from build123d import *

# Parameters (mm, degrees)
SKETCH_1_W               = 20
SKETCH_1_H               = 20
EXTRUDE_1_DEPTH          = 150
SKETCH_3_R               = 3.2
CUT_EXTRUDE_2_DEPTH      = 18
SKETCH_4_R               = 3.1
CUT_EXTRUDE_3_DEPTH      = 3.2
MIRROR_3_COPY_1_SKETCH_R = 3.1
MIRROR_3_COPY_1_DEPTH    = 3.2
MIRROR_4_COPY_1_SKETCH_R = 3.2
MIRROR_4_COPY_1_DEPTH    = 18
MIRROR_4_COPY_2_SKETCH_R = 3.1
MIRROR_4_COPY_2_DEPTH    = 3.2
MIRROR_4_COPY_3_SKETCH_R = 3.1
MIRROR_4_COPY_3_DEPTH    = 3.2
MIRROR_4_COPY_4_SKETCH_R = 3.1
MIRROR_4_COPY_4_DEPTH    = 3.2


with BuildPart() as part:
    # ｽｹｯﾁ1 → ﾎﾞｽ - 押し出し1 (new body)
    with BuildSketch(Plane.XY):
        Rectangle(SKETCH_1_W, SKETCH_1_H)
    extrude_1 = extrude(amount=EXTRUDE_1_DEPTH)

    # ｽｹｯﾁ3 → ｶｯﾄ - 押し出し2 (cut)
    with BuildSketch(Plane(origin=(0, 10, 0), x_dir=(1, 0, 0), z_dir=(0, 1, 0))):
        with Locations(Location((5, -5, 0), (0, 0, 270))):
            Circle(SKETCH_3_R)
    cut_extrude_2 = extrude(amount=-CUT_EXTRUDE_2_DEPTH, mode=Mode.SUBTRACT)

    # ﾐﾗｰ1: ｶｯﾄ - 押し出し2 across plane
    add(cut_extrude_2.mirror(Plane(origin=(0, 0, 0), x_dir=(0, 0, 1), z_dir=(1, 0, 0))), mode=Mode.SUBTRACT)

    # ｽｹｯﾁ4 → ｶｯﾄ - 押し出し3 (cut)
    with BuildSketch(Plane.XY.offset(150)):
        with Locations((5, 5)):
            Circle(SKETCH_4_R)
    cut_extrude_3 = extrude(amount=-CUT_EXTRUDE_3_DEPTH, mode=Mode.SUBTRACT)

    # ﾐﾗｰ2: ｶｯﾄ - 押し出し3 across plane
    add(cut_extrude_3.mirror(Plane.ZX), mode=Mode.SUBTRACT)

    # ﾐﾗｰ3: ｶｯﾄ - 押し出し3 across plane
    add(cut_extrude_3.mirror(Plane(origin=(0, 0, 0), x_dir=(0, 0, 1), z_dir=(1, 0, 0))), mode=Mode.SUBTRACT)

    # ﾐﾗｰ3 copy 1 sketch → ﾐﾗｰ3 copy 1 (cut)
    with BuildSketch(Plane(origin=(0, 0, 150), x_dir=(-1, 0, 0), z_dir=(0, 0, 1))):
        with Locations((5, 5)):
            Circle(MIRROR_3_COPY_1_SKETCH_R)
    extrude(amount=-MIRROR_3_COPY_1_DEPTH, mode=Mode.SUBTRACT)

    # ﾐﾗｰ4: ﾎﾞｽ - 押し出し1, ｶｯﾄ - 押し出し2, ｶｯﾄ - 押し出し3 across plane
    add(extrude_1.mirror(Plane(origin=(-10, 10, 150), x_dir=(0, 0, 1), z_dir=(1, 0, 0))))
    add(cut_extrude_2.mirror(Plane(origin=(-10, 10, 150), x_dir=(0, 0, 1), z_dir=(1, 0, 0))), mode=Mode.SUBTRACT)
    add(cut_extrude_3.mirror(Plane(origin=(-10, 10, 150), x_dir=(0, 0, 1), z_dir=(1, 0, 0))), mode=Mode.SUBTRACT)

    # ﾐﾗｰ4 copy 1 sketch → ﾐﾗｰ4 copy 1 (cut)
    with BuildSketch(Plane(origin=(-20, 10, 0), x_dir=(1, 0, 0), z_dir=(0, 1, 0))):
        with Locations(Location((5, -5, 0), (0, 0, 270))):
            Circle(MIRROR_4_COPY_1_SKETCH_R)
    extrude(amount=-MIRROR_4_COPY_1_DEPTH, mode=Mode.SUBTRACT)

    # ﾐﾗｰ4 copy 2 sketch → ﾐﾗｰ4 copy 2 (cut)
    with BuildSketch(Plane(origin=(-20, 0, 150), x_dir=(-1, 0, 0), z_dir=(0, 0, 1))):
        with Locations((5, 5)):
            Circle(MIRROR_4_COPY_2_SKETCH_R)
    extrude(amount=-MIRROR_4_COPY_2_DEPTH, mode=Mode.SUBTRACT)

    # ﾐﾗｰ4 copy 3 sketch → ﾐﾗｰ4 copy 3 (cut)
    with BuildSketch(Plane(origin=(-20, 0, 150), x_dir=(1, 0, 0), z_dir=(0, 0, 1))):
        with Locations((5, 5)):
            Circle(MIRROR_4_COPY_3_SKETCH_R)
    extrude(amount=-MIRROR_4_COPY_3_DEPTH, mode=Mode.SUBTRACT)

    # ﾐﾗｰ4 copy 4 sketch → ﾐﾗｰ4 copy 4 (cut)
    with BuildSketch(Plane(origin=(-20, 0, 150), x_dir=(1, 0, 0), z_dir=(0, 0, 1))):
        with Locations((5, -5)):
            Circle(MIRROR_4_COPY_4_SKETCH_R)
    extrude(amount=-MIRROR_4_COPY_4_DEPTH, mode=Mode.SUBTRACT)


solid = part.part
Input: part model. Units: mm. Frame: model coordinates. A direction names the side the tool comes from. Coordinates: 2 decimals unless noted, no trailing zeros. Loops run counter-clockwise (first coordinate to the right, second up) from the corner with the lowest first, then second, coordinate; pieces in that order, holes last.
Q1. Set-up query: faces 1 (the face through (-5, -8, 5)), 2 (the face through (-22.54, -3.114, 148.422)), 3 (the face through (-10, 0, 150)). Return all of +Z, -Z, +X, -X, +Y, -Y with unobstructed straight access to the full face (end or side cutting, diameter ignored); none if empty.
Q2. Draft query along Z for faces 4 (the face through (-10, -10, 74)), 5 (the face through (3.053, 1.126, 2.461)), 6 (the face through (5, -5, 146.8)). Return one class per face: +Z half, -Z half, draft (parallel to the pull), parting line (faces both ways), or undercut.
Q3. Cut plane A-A (z = 5). Output: boundary loops of the cut face in (x, y).
Q4. Material intervals for line 1 (Y direction, x = -15, z = 149.1); line 2 (X direction, y = 1, z = 5); line 3 (Z direction, x = -5.5, y = 8.25), sorted ascending.
Q5. Cut plane B-B (y = -5). Output: boundary loops of the cut face in (x, z).
Q6. Cut plane C-C (x = -15). Output: boundary loops of the cut face in (y, z).
Q7. Contact query for flat-ended pins moving along their axis: pin 1 (5 mm diameter, centred on x = -25, y = 5, fed in from +Z); pin 2 (8.5 mm diameter, centred on x = 5, z = 5, fed in from +Y); pin 3 (1.9 mm diameter, centred on x = -3.5, z = 4, fed in from +Y). Output: stop coordinate, or through.
Working result:
1. face 1: +Y
1. face 2: +Z
1. face 3: +Z, +X, -X, +Y, -Y
2. face 4: draft
2. face 5: undercut
2. face 6: +Z half
3. outline: (-30, -10) - (10, -10) - (10, 10) - (8.2, 10) - (8.2, -8) - (1.8, -8) - (1.8, 10) - (-1.8, 10) - (-1.8, -8) - (-8.2, -8) - (-8.2, 10) - (-11.8, 10) - (-11.8, -8) - (-18.2, -8) - (-18.2, 10) - (-21.8, 10) - (-21.8, -8) - (-28.2, -8) - (-28.2, 10) - (-30, 10) - close
4. line 1: y = -10 to -8.1, -1.9 to 1.9, 8.1 to 10
4. line 2: x = -30 to -28.2, -21.8 to -18.2, -11.8 to -8.2, -1.8 to 1.8, 8.2 to 10
4. line 3: z = 0 to 1.84, 8.16 to 150
5. outline: (-30, 0) - (10, 0) - (10, 150) - (8.1, 150) - (8.1, 146.8) - (1.9, 146.8) - (1.9, 150) - (-1.9, 150) - (-1.9, 146.8) - (-8.1, 146.8) - (-8.1, 150) - (-11.9, 150) - (-11.9, 146.8) - (-18.1, 146.8) - (-18.1, 150) - (-21.9, 150) - (-21.9, 146.8) - (-28.1, 146.8) - (-28.1, 150) - (-30, 150) - close; hole circle Ø6.4 at (-25, 5); hole circle Ø6.4 at (-15, 5); hole circle Ø6.4 at (-5, 5); hole circle Ø6.4 at (5, 5)
6. outline: (-10, 0) - (10, 0) - (10, 1.8) - (-8, 1.8) - (-8, 8.2) - (10, 8.2) - (10, 150) - (8.1, 150) - (8.1, 146.8) - (1.9, 146.8) - (1.9, 150) - (-1.9, 150) - (-1.9, 146.8) - (-8.1, 146.8) - (-8.1, 150) - (-10, 150) - close
7. pin 1: stops at z = 146.8
7. pin 2: stops at y = 10
7. pin 3: stops at y = -8
